Could you check a few things on this model? Use its own coordinates, in mm. Face numbers are marked on the shaded views. Round coordinates to 2 decimals unless told otherwise and drop trailing zeros. Write each loop counter-clockwise with the first axis right and the second up, starting at its lowest first coordinate (ties: lowest second). Pieces come first, ordered by that corner, then holes. Notation, with made-up numbers: (74.25, 48.5) -> (89.25, 48.5) arc R15 cw to (89.25, 71.5) -> close; hole circle Ø9 at (89, 46). An arc over 180 degrees is marked (long way). Answer as CSV lines item,"result". Start each with the question number.
Q1. If we mould it in two halves opening along X, with no side actions, what happens to the marked faces 1, 2 and 3? For each: pulls with the +X half, pulls with the -X half, needs draft (parallel to the pull), parting line crosses it, or undercut.
Q2. Imagine slicing it at D-D on z = -21. Please give me the cut outline in (x, y).
Q3. Imagine slicing it at C-C on x = -6. Please give me the cut outline in (y, z), and give its area (3 significant figures).
Q4. Imagine slicing it at B-B on z = -25.4. Please give me the cut outline in (x, y).
Q5. If I drill on line 1 (X direction, y = 1.6, z = -25.4); line 2 (X direction, y = 0.55, z = -27.5); line 3 (Z direction, x = -8, y = 2.6), over which ranges is the centre line in solid material (lowest first)? Write a range as [from, to].
Q6. Will these pins go through, and if not, where does the flat tip stop? pin 1 Ø1 at (y, z) = (4, -11.5) entering from +X; pin 2 Ø2 at (x, y) = (9, 3) entering from +Z; pin 3 Ø2 at (y, z) = (1.5, -10.5) entering from -X.
Q7. Imagine slicing it at A-A on x = 0. Please give me the cut outline in (y, z) (1 decimal).
from build123d import *

# Parameters (mm, degrees)
SKETCH1_R            = 9.525
BOSS_EXTRUDE1_DEPTH  = 4.7625
FILLET1_R            = 0.79375
M6_CLEARANCE_HOLE1_D = 6.6


with BuildPart() as part:
    # Sketch1 → Boss-Extrude1 (new body)
    with BuildSketch(Plane(origin=(0, 0, 0), x_dir=(1, 0, 0), z_dir=(0, 1, 0))):
        with Locations((0, 25.4)):
            Circle(SKETCH1_R)
        with BuildLine():
            Line((-9.450292964208833, 26.590625), (-12.60039061894511, 1.5874999999999988))
            ThreePointArc((-12.60039061894511, 1.5875000000000075), (6.42e-15, 12.699999999999998), (12.600390618945111, 1.587499999999999))
            Line((12.60039061894511, 1.5874999999999988), (9.450292964208833, 26.590625))
            ThreePointArc((9.450292964208835, 26.590625), (9.506304894229123, 25.996483241973674), (9.525, 25.4))
            ThreePointArc((9.525, 25.399999999999995), (-0.5964832419736728, 15.893695105770876), (-9.450292964208835, 26.590625))
        make_face()
    extrude(amount=BOSS_EXTRUDE1_DEPTH)

    # Fillet1
    fillet1_edges = [part.edges().sort_by_distance(p)[0] for p in [
        (-12.60039061894511, 2.38125, -1.587500000000003),
    ]]
    fillet(fillet1_edges, radius=FILLET1_R)
    fillet1_2_edges = [part.edges().sort_by_distance(p)[0] for p in [
        (12.60039061894511, 2.38125, -1.5874999999999981),
    ]]
    fillet(fillet1_2_edges, radius=FILLET1_R)

    # M6 Clearance Hole1 (through all)
    with Locations(Plane(origin=(0, 4.7625, 0), x_dir=(1, 0, 0), z_dir=(0, 1, 0))):
        with Locations((0, 25.4)):
            Hole(M6_CLEARANCE_HOLE1_D / 2)


solid = part.part
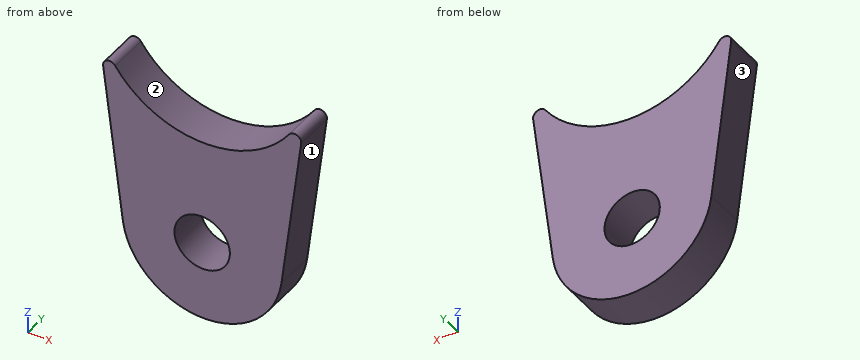
Checks:
1,face 1,"pulls with the +X half"
1,face 2,"undercut"
1,face 3,"pulls with the -X half"
2,outline,"(-10.15, 0) -> (10.15, 0) -> (10.15, 4.76) -> (-10.15, 4.76) -> close"
3,outline,"(0, -32.8) -> (4.76, -32.8) -> (4.76, -11.19) -> (0, -11.19) -> close"
3,area,"103 mm^2"
4,outline,"(-9.6, 0) -> (-3.3, 0) -> (-3.3, 4.76) -> (-9.6, 4.76) -> close; (3.3, 0) -> (9.6, 0) -> (9.6, 4.76) -> (3.3, 4.76) -> close"
5,line 1,"[-9.6, -3.3], [3.3, 9.6]"
5,line 2,"[-9.29, -2.55], [2.55, 9.29]"
5,line 3,"[-30.57, -9.86]"
6,pin 1,"x = 11.41"
6,pin 2,"z = -7.83"
6,pin 3,"x = -11.6"
7,outline,"(0, -34.9) -> (4.8, -34.9) -> (4.8, -28.7) -> (0, -28.7) -> close; (0, -22.1) -> (4.8, -22.1) -> (4.8, -12.7) -> (0, -12.7) -> close"
